```python
from build123d import *

# Parameters (mm, degrees)
F0_W     = 156.882346
F0_H     = 84.193528
F0_W_2   = 141.194134
F0_H_2   = 67.982354
F1_DEPTH = 101.6
F2_W     = 79.92284
F2_H     = 42.2275
F3_DEPTH = 190.754
F5_D     = 25.4


with BuildPart() as f1:
    # F0 (on Top) → F1 (new body)
    with BuildSketch(Plane.XY):
        Rectangle(F0_W, F0_H)
        Rectangle(F0_W_2, F0_H_2, mode=Mode.SUBTRACT)
    extrude(amount=F1_DEPTH)

    # F2 (on face) → F3 (cut, symmetric)
    with BuildSketch(Plane.XZ.offset(42.096764)):
        with Locations((0, 80.48625)):
            Rectangle(F2_W, F2_H)
    extrude(amount=F3_DEPTH, both=True, mode=Mode.SUBTRACT)

    # F5 (through all)
    with Locations(Plane.YZ.offset(78.441173)):
        with Locations((0, 50.8)):
            Hole(F5_D / 2)


solid = f1.part
```
For this review, take the finished solid that the model builds, in its own axes (mm). A direction names the side the tool comes from. Round coordinates to 2 decimals unless told otherwise and drop trailing zeros. Write each loop counter-clockwise with the first axis right and the second up, starting at its lowest first coordinate (ties: lowest second). Pieces come first, ordered by that corner, then holes. Notation, with made-up numbers: (17.5, 36) -> (42.5, 36) arc R15 ccw to (42.5, 52) -> close; hole circle Ø4 at (1, 20). An arc over 180 degrees is marked (long way). One line per question, with ' | ' between items. Start each with the question number.
(1) Mouldability with a two-part tool opening along Y and no side actions: class faces 4 (the face through (-1, 42.097, 39)), 5 (the face through (-74.574, -5.86, 39.533)), 6 (the face through (-0.4, 34.5, 0)), 7 (the face through (-1, -42.097, 39)) as released by +Y, released by -Y, zero draft, split by the parting line, or undercut.
(2) Add section B-B, the plane y = -23. Write out the cut boundary in (x, z).
(3) Insertion check: P1, Ø9, axis at x = 16, y = 37.5, coming from the +Z side. The pin has a flat end and moves straight along its axis. Give the tip position at first contact, or say it passes through.
(4) Add section D-D, the plane y = 0. Write out the cut boundary in (x, z), plus the area to 3 significant figures.
(5) Add section A-A, the plane x = 19.5. Write out the cut boundary in (y, z), plus the area to 4 significant figures.
(6) Add section C-C, the plane z = 67. Write out the cut boundary in (x, y), plus the area to 3 significant figures.
(7) For line 1 along Y through (x, z) = (60.5, 31.5); line 2 along Z through (x, y) = (-74, 0); line 3 along X through (y, z) = (-17.5, 21.5), list the stretches that pass through material, from the lowest coordinate up. Write a range as from..to.
(8) Tool access review of faces 1 (the face through (72, 1, 101.6)), 2 (the face through (-39.961, -38, 80)), 3 (the face through (-1, 33.991, 39)): name each direction out of +Z, -Z, +X, -X, +Y, -Y from which nothing blocks a thin tool from reaching the whole face with its end or side.
Answer list:
1) face 4: released by +Y | face 5: undercut | face 6: zero draft | face 7: released by -Y
2) outline: (-78.44, 0) -> (-70.6, 0) -> (-70.6, 101.6) -> (-78.44, 101.6) -> close; (70.6, 0) -> (78.44, 0) -> (78.44, 101.6) -> (70.6, 101.6) -> close
3) P1: z = 59.37
4) outline: (-78.44, 0) -> (-70.6, 0) -> (-70.6, 38.1) -> (-78.44, 38.1) -> close; (-78.44, 63.5) -> (-70.6, 63.5) -> (-70.6, 101.6) -> (-78.44, 101.6) -> close; (70.6, 0) -> (78.44, 0) -> (78.44, 38.1) -> (70.6, 38.1) -> close; (70.6, 63.5) -> (78.44, 63.5) -> (78.44, 101.6) -> (70.6, 101.6) -> close | area: 1,200 mm²
5) outline: (-42.1, 0) -> (-33.99, 0) -> (-33.99, 59.37) -> (-42.1, 59.37) -> close; (33.99, 0) -> (42.1, 0) -> (42.1, 59.37) -> (33.99, 59.37) -> close | area: 962.5 mm²
6) outline: (-78.44, -42.1) -> (-39.96, -42.1) -> (-39.96, -33.99) -> (-70.6, -33.99) -> (-70.6, 33.99) -> (-39.96, 33.99) -> (-39.96, 42.1) -> (-78.44, 42.1) -> close; (39.96, -42.1) -> (78.44, -42.1) -> (78.44, 42.1) -> (39.96, 42.1) -> (39.96, 33.99) -> (70.6, 33.99) -> (70.6, -33.99) -> (39.96, -33.99) -> close | area: 2,310 mm²
7) line 1: -42.1..-33.99, 33.99..42.1 | line 2: 0..38.1, 63.5..101.6 | line 3: -78.44..-70.6, 70.6..78.44
8) face 1: +Z, +X, -X, +Y, -Y | face 2: +Z, +Y, -Y | face 3: +Z, -Z
